Can you work these out from the model? Positions are in its coordinate system, mm. Give positions to 0.01 mm unless a question says otherwise; leave off trailing zeros. Write each loop counter-clockwise with the first axis right and the second up, starting at its lowest first coordinate (ties: lowest second). Pieces come first, ordered by that corner, then holes.
1. Suppose I cut it at B-B (y = 11). Please give me the cut outline in (x, z) (3 decimals), and give its area (3 significant figures).
2. Suppose I cut it at C-C (z = 0.95). Give the number of separate pieces and of enclosed holes in the cut face, and give its area (3 significant figures).
3. If I drill on probe 1 along Y at (x, z) = (-8.5, 0.7) (3 decimals); probe 2 along Y at (x, z) = (11, -0.55) (3 decimals); probe 3 along Y at (x, z) = (9.75, 0.15), over which ranges is the centre line in solid material (lowest first)?
4. I'm going to push flat-ended pins straight in: pin 1 (3.5 mm diameter, centred on x = -11, y = 11, fed in from +Z); pin 2 (1.8 mm diameter, centred on x = 11, y = 11, fed in from -Z). Where does each tip first touch, or does it pass through?
5. Suppose I cut it at A-A (x = -8.5). Please give me the cut outline in (y, z) (3 decimals), and give its area (3 significant figures).
6. Suppose I cut it at D-D (y = -21.5). Please give me the cut outline in (x, z).
```python
from build123d import *

# Parameters (mm, degrees)
SKETCH_1_W          = 30
SKETCH_1_H          = 30
SKETCH_1_W_2        = 25
EXTRUDE_1_DEPTH     = 1.5
EXTRUDE_2_DEPTH     = 3
SKETCH_5_R          = 1.505
CUT_EXTRUDE_2_DEPTH = 3
SKETCH_3_R          = 1.505
CUT_EXTRUDE_1_DEPTH = 3
FILLET_1_R          = 2


with BuildPart() as part:
    # 草图1 → 凸台-拉伸1 (new, symmetric)
    with BuildSketch(Plane.XY):
        Rectangle(SKETCH_1_W, SKETCH_1_H)
        with Locations((0, -30)):
            Rectangle(SKETCH_1_W_2, SKETCH_1_H)
    extrude(amount=EXTRUDE_1_DEPTH, both=True)

    # 草图2 → 凸台-拉伸2 (add)
    with BuildSketch(Plane.XY.offset(1.5)):
        Polygon((-15, -15), (-12.5, -45), (12.5, -45), (15, -15), align=None)
    extrude(amount=-EXTRUDE_2_DEPTH)

    # 草图5 → 切除-拉伸2 (cut)
    with BuildSketch(Plane(origin=(0, 0, -1.5), x_dir=(-1, 0, 0), z_dir=(0, 0, -1))):
        with Locations((-8.5, -19)):
            Circle(SKETCH_5_R)
        with Locations((8.5, -19)):
            Circle(SKETCH_5_R)
        with Locations((-8.5, -41)):
            Circle(SKETCH_5_R)
        with Locations((8.5, -41)):
            Circle(SKETCH_5_R)
    extrude(amount=-CUT_EXTRUDE_2_DEPTH, mode=Mode.SUBTRACT)

    # 草图3 → 切除-拉伸1 (cut)
    with BuildSketch(Plane(origin=(0, 0, -1.5), x_dir=(-1, 0, 0), z_dir=(0, 0, -1))):
        with Locations((-11, 11)):
            Circle(SKETCH_3_R)
        with Locations((11, 11)):
            Circle(SKETCH_3_R)
        with Locations((-11, -11)):
            Circle(SKETCH_3_R)
        with Locations((11, -11)):
            Circle(SKETCH_3_R)
    extrude(amount=-CUT_EXTRUDE_1_DEPTH, mode=Mode.SUBTRACT)

    # 圆角1
    # the kernel refuses this fillet: 2 mm, written as the material it takes off along each edge
    with BuildSketch(Plane(origin=(-15, -15, 1.707972894), x_dir=(0, 1, 0), z_dir=(0, 0, -1)), Plane(origin=(15, -15, -1.707972894), x_dir=(0, 1, 0), z_dir=(0, 0, 1))) as fillet_1_piece_1:
        with BuildLine():
            CenterArc((FILLET_1_R * 0.0415945787923, FILLET_1_R), FILLET_1_R, 265.236358309, 4.763641691)
            Line((-FILLET_1_R * 0.0414509010614, FILLET_1_R * 0.00345424175512), (0, 0))
            Line((0, 0), (FILLET_1_R * 0.0415945787923, 0))
        make_face()
    extrude(amount=3.415945788, mode=Mode.SUBTRACT)
    with BuildSketch(Plane(origin=(-15, 15, 6.5), x_dir=(0, -1, 0), z_dir=(0, 0, -1))) as fillet_1_piece_2:
        with BuildLine():
            CenterArc((FILLET_1_R, -FILLET_1_R), FILLET_1_R, 90, 90)
            Line((0, -FILLET_1_R), (0, 0))
            Line((0, 0), (FILLET_1_R, 0))
        make_face()
    extrude(amount=13, mode=Mode.SUBTRACT)
    with BuildSketch(Plane(origin=(15, 15, -6.5), x_dir=(-1, 0, 0), z_dir=(0, 0, 1))) as fillet_1_piece_3:
        with BuildLine():
            CenterArc((FILLET_1_R, FILLET_1_R), FILLET_1_R, 180, 90)
            Line((0, FILLET_1_R), (0, 0))
            Line((0, 0), (FILLET_1_R, 0))
        make_face()
    extrude(amount=13, mode=Mode.SUBTRACT)
    with BuildSketch(Plane(origin=(12.5, -45, 6.100664408), x_dir=(-1, 0, 0), z_dir=(0, 0, -1))) as fillet_1_piece_4:
        with BuildLine():
            CenterArc((FILLET_1_R * 0.920132881566, FILLET_1_R), FILLET_1_R, 184.763641691, 85.236358309)
            Line((-FILLET_1_R * 0.0764128766789, FILLET_1_R * 0.916954520146), (0, 0))
            Line((0, 0), (FILLET_1_R * 0.920132881566, 0))
        make_face()
    extrude(amount=12.201328816, mode=Mode.SUBTRACT)
    with BuildSketch(Plane(origin=(-12.5, -45, -6.100664408), x_dir=(-0.08304547985374029, 0.9965457582448797, 0), z_dir=(0, 0, 1))) as fillet_1_piece_5:
        with BuildLine():
            CenterArc((FILLET_1_R * 0.920132881566, -FILLET_1_R), FILLET_1_R, 90, 85.236358309)
            Line((-FILLET_1_R * 0.0764128766789, -FILLET_1_R * 0.916954520146), (0, 0))
            Line((0, 0), (FILLET_1_R * 0.920132881566, 0))
        make_face()
    extrude(amount=12.201328816, mode=Mode.SUBTRACT)


solid = part.part
```
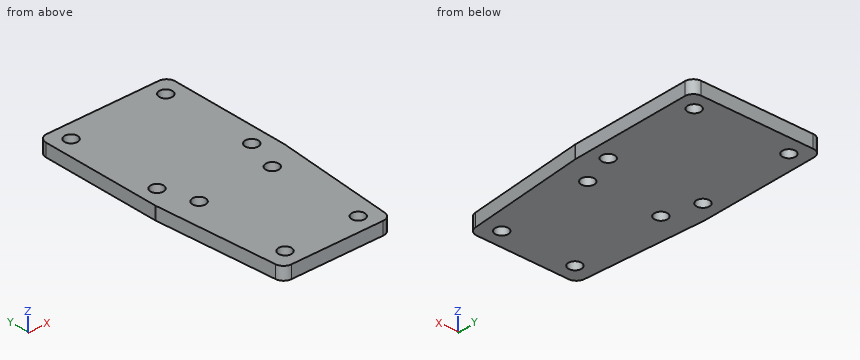
Checks:
1. outline: (-15, -1.5) - (-12.505, -1.5) - (-12.505, 1.5) - (-15, 1.5) - close; (-9.495, -1.5) - (9.495, -1.5) - (9.495, 1.5) - (-9.495, 1.5) - close; (12.505, -1.5) - (15, -1.5) - (15, 1.5) - (12.505, 1.5) - close
1. area: 71.9 mm2
2. separate pieces: 1
2. enclosed holes: 8
2. area: 1,660 mm2
3. probe 1: y = -45 to -42.505, -39.495 to -20.505, -17.495 to 15
3. probe 2: y = -44.971 to -12.505, -9.495 to 9.495, 12.505 to 15
3. probe 3: y = -45 to -41.84, -40.16 to -19.84, -18.16 to -11.84, -10.16 to 10.16, 11.84 to 15
4. pin 1: stops at z = 1.5
4. pin 2: passes through
5. outline: (-45, -1.5) - (-42.505, -1.5) - (-42.505, 1.5) - (-45, 1.5) - close; (-39.495, -1.5) - (-20.505, -1.5) - (-20.505, 1.5) - (-39.495, 1.5) - close; (-17.495, -1.5) - (15, -1.5) - (15, 1.5) - (-17.495, 1.5) - close
5. area: 162 mm2
6. outline: (-14.46, -1.5) - (14.46, -1.5) - (14.46, 1.5) - (-14.46, 1.5) - close
